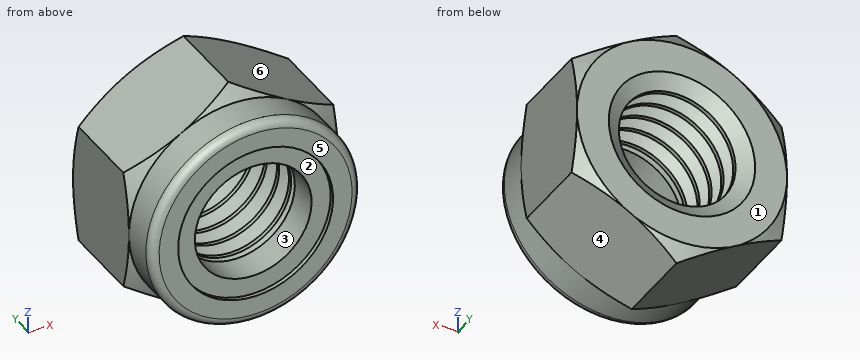
```python
from build123d import *
from build123d.topology import SkipClean

# Parameters (mm, degrees)
SKETCH1_R           = 3.4925
BOSS_EXTRUDE1_DEPTH = 5.9436
BOSS_EXTRUDE2_START = 2.3114
SKETCH2_R           = 6.280156421
SKETCH2_R_2         = 3.4925
BOSS_EXTRUDE2_DEPTH = 2.3114
FILLET2_R           = 0.508
SKETCH4_R           = 4.6355
SKETCH4_R_2         = 3.4925
CUT_EXTRUDE1_DEPTH  = 0.254
SKETCH6_R           = 4.6355
SKETCH6_R_2         = 3.4925
BOSS_EXTRUDE3_DEPTH = 1.778


with BuildPart() as part:
    # Sketch1 → Boss-Extrude1 (new body)
    with BuildSketch(Plane(origin=(0, 0, 0), x_dir=(1, 0, 0), z_dir=(0, 1, 0))):
        Polygon((0, -7.2517), (6.280156421, -3.62585), (6.280156421, 3.62585), (0, 7.2517), (-6.280156421, 3.62585), (-6.280156421, -3.62585), align=None)
        with Locations(Location((0, 0, 0), (0, 0, 270))):
            Circle(SKETCH1_R, mode=Mode.SUBTRACT)
    extrude(amount=BOSS_EXTRUDE1_DEPTH)

    # Sketch2 → Boss-Extrude2 (add)
    with SkipClean():  # the faces are left unmerged after this step: merging them gives an invalid solid
        with BuildSketch(Plane.XZ.offset(BOSS_EXTRUDE2_START)):
            with Locations(Location((0, 0, 0), (0, 0, 120))):
                Circle(SKETCH2_R)
            with Locations(Location((0, 0, 0), (0, 0, 270))):
                Circle(SKETCH2_R_2, mode=Mode.SUBTRACT)
        extrude(amount=-BOSS_EXTRUDE2_DEPTH)

    # Fillet2
    fillet2_edges = [part.edges().sort_by_distance(p)[0] for p in [
        (3.14007821, -2.3114, -5.438775),
    ]]
    fillet(fillet2_edges, radius=FILLET2_R)

    # Sketch3 → Cut-Revolve1 (revolve, cut)
    with BuildSketch(Plane(origin=(0, 0, 0), x_dir=(0, 0, -1), z_dir=(1, 0, 0)), mode=Mode.PRIVATE) as cut_revolve1_sk:
        Polygon((-7.2517, 0.593112632), (-7.2517, 0), (-6.280156421, 0), align=None)
        Polygon((-6.280156421, 5.9436), (-7.2517, 5.9436), (-7.2517, 5.355420001), align=None)
        Polygon((-3.391632963, 6.5151), (-4.3815, 5.9436), (-3.294472118, 5.31600416), align=None)
        Polygon((-3.391632963, 5.2451), (-4.3815, 4.6736), (-3.294472118, 4.04600416), align=None)
        Polygon((-3.391632963, 3.9751), (-4.3815, 3.4036), (-3.294472118, 2.77600416), align=None)
        Polygon((-3.391632963, 2.7051), (-4.3815, 2.1336), (-3.294472118, 1.50600416), align=None)
        Polygon((-3.391632963, 1.4351), (-4.3815, 0.8636), (-3.294472118, 0.23600416), align=None)
        Polygon((-3.391632963, 0.1651), (-4.3815, -0.4064), (-3.294472118, -1.03399584), align=None)
        Polygon((-3.391632963, -1.1049), (-4.3815, -1.6764), (-3.294472118, -2.30399584), align=None)
    revolve(cut_revolve1_sk.sketch.rotate(Axis((0, 0, 0), (0, 1, 0)), 180), axis=Axis((0, 0, 0), (0, 1, 0)), mode=Mode.SUBTRACT)

    # Sketch4 → Cut-Extrude1 (cut)
    with BuildSketch(Plane.XZ.offset(2.3114)):
        with Locations(Location((0, 0, 0), (0, 0, 270))):
            Circle(SKETCH4_R)
        with Locations(Location((0, 0, 0), (0, 0, 270))):
            Circle(SKETCH4_R_2, mode=Mode.SUBTRACT)
    extrude(amount=-CUT_EXTRUDE1_DEPTH, mode=Mode.SUBTRACT)

    # Sketch6 → Boss-Extrude3 (add)
    with BuildSketch(Plane.XZ.offset(2.0574)):
        with Locations(Location((0, 0, 0), (0, 0, 270))):
            Circle(SKETCH6_R)
        with Locations(Location((0, 0, 0), (0, 0, 270))):
            Circle(SKETCH6_R_2, mode=Mode.SUBTRACT)
    extrude(amount=-BOSS_EXTRUDE3_DEPTH)


solid = part.part
```
The model under review builds one solid part; all positions refer to its coordinate system, in mm. Face numbers are marked on the shaded views. A direction names the side the tool comes from. Round coordinates to 2 decimals unless told otherwise and drop trailing zeros. Loops run counter-clockwise (first coordinate to the right, second up) from the corner with the lowest first, then second, coordinate; pieces in that order, holes last. Notation, with made-up numbers: (-23.75, 52.5) -> (28.25, 52.5) arc R22 ccw to (28.25, 70.5) -> close; hole circle Ø5 at (4, 0). An arc over 180 degrees is marked (long way). Answer as a JSON object with one key per item and string values. Group by question number.
1) We need section A-A on y = -1.5. Write out the cut boundary in (x, z) (1 decimal).
2) For the marked faces 1 and 2, list the 3-axis set-ups (+Z, -Z, +X, -X, +Y, -Y) from which the entire face can be reached by the end or side of a thin tool; tool diameter is ignored.
3) For pin 1 Ø1.5 at (x, z) = (-5, -5) entering from +Y; pin 2 Ø2 at (x, y) = (-3.5, 0.5) entering from -Z; pin 3 Ø4.5 at (x, z) = (0.5, -2) entering from -Y, all flat-tipped, find the tip position at first contact; note any pin that passes through.
4) For line 1 (X direction, y = 0.2, z = 0); line 2 (X direction, y = 5.5, z = 0); line 3 (Y direction, x = 4.75, z = -4), list the stretches that pass through material, from the lowest coordinate up. Write a range as [from, to].
5) Mouldability with a two-part tool opening along Z and no side actions: class the marked faces 3, 4, 5 and 6 as released by +Z, released by -Z, zero draft, split by the parting line, or undercut.
Result set:
{
 "1": {"outline": "circle Ø12.6 at (0, 0); hole circle Ø7 at (0, 0)"},
 "2": {"face 1": "+Z, -Z, +X, -X, +Y", "face 2": "-Y"},
 "3": {"pin 1": "y = 5.92", "pin 2": "z = -5.81", "pin 3": "y = -2.06"},
 "4": {"line 1": "[-6.28, -3.49], [3.49, 6.28]", "line 2": "[-6.28, -3.61], [3.61, 6.28]", "line 3": "[-2.06, 5.94]"},
 "5": {"face 3": "undercut", "face 4": "released by -Z", "face 5": "zero draft", "face 6": "released by +Z"}
}
